from build123d import *

# Parameters (mm, degrees)
CUT_EXTRUDE1_START = -7
CUT_EXTRUDE1_DEPTH = 6


with BuildPart() as part:
    # Sketch3 → Revolve1 (revolve)
    with BuildSketch(Plane.XY, mode=Mode.PRIVATE) as revolve1_sk:
        Polygon((-7, 1.6), (6, 1.6), (6, 12), (15, 12), (15, 16), (-14, 16), (-14, 18), (-16, 18), (-16, 13), (-7, 13), align=None)
    revolve(revolve1_sk.sketch.rotate(Axis((0, 0, 0), (1, 0, 0)), 90), axis=Axis((0, 0, 0), (1, 0, 0)))

    # Sketch4 → Cut-Extrude1 (cut)
    with BuildSketch(Plane(origin=(0, 0, 0), x_dir=(0, 0, -1), z_dir=(1, 0, 0)).offset(CUT_EXTRUDE1_START)):
        Polygon((3.608439182, 6.25), (-3.608439182, 6.25), (-7.216878365, 0), (-3.608439182, -6.25), (3.608439182, -6.25), (7.216878365, 0), align=None)
    extrude(amount=CUT_EXTRUDE1_DEPTH, mode=Mode.SUBTRACT)


solid = part.part
Model file for the job. Use its own axes, mm. A direction names the side the tool comes from. Give positions to 0.01 mm unless a question says otherwise; leave off trailing zeros. Loops run counter-clockwise (first coordinate to the right, second up) from the corner with the lowest first, then second, coordinate; pieces in that order, holes last.
Item 1: Slice it at D-D (y = -5.5). Write the cut outline in (x, z), plus the area to 3 significant figures.
Check values:
outline: (-16, -17.14) - (-14, -17.14) - (-14, -15.02) - (15, -15.02) - (15, -10.67) - (6, -10.67) - (6, 10.67) - (15, 10.67) - (15, 15.02) - (-14, 15.02) - (-14, 17.14) - (-16, 17.14) - (-16, 11.78) - (-7, 11.78) - (-7, 4.04) - (-1, 4.04) - (-1, -4.04) - (-7, -4.04) - (-7, -11.78) - (-16, -11.78) - close
area: 488 mm2
Item 2: Slice it at B-B (x = -9.5). Write the cut outline in (y, z).
Check values:
outline: circle Ø32 at (0, 0); hole circle Ø26 at (0, 0)
Item 3: Slice it at A-A (z = 0). Write the cut outline in (x, y), plus the area to 3 significant figures.
Check values:
outline: (-16, -18) - (-14, -18) - (-14, -16) - (15, -16) - (15, -12) - (6, -12) - (6, -1.6) - (-1, -1.6) - (-1, -6.25) - (-7, -6.25) - (-7, -13) - (-16, -13) - close; (-16, 13) - (-7, 13) - (-7, 6.25) - (-1, 6.25) - (-1, 1.6) - (6, 1.6) - (6, 12) - (15, 12) - (15, 16) - (-14, 16) - (-14, 18) - (-16, 18) - close
area: 453 mm2
Item 4: Drill centre lines: line 1 along Y through (x, z) = (11, 0); line 2 along Y through (x, z) = (-12, 0); line 3 along X through (y, z) = (6.5, -10.5). Where is each one in solid material? Low to high.
Check values:
line 1: y = -16 to -12, 12 to 16
line 2: y = -16 to -13, 13 to 16
line 3: x = -7 to 15
Item 5: Mould opens along Z. For faces 4 (the face through (-7, -3, 6)), 5 (the face through (6, 0, -2)), 6 (the face through (-15.014, -12.165, -13.267)), 7 (the face through (-14, 11, 12)) say: +Z half, -Z half, draft (parallel to the pull), parting line (faces both ways), or undercut.
Check values:
face 4: undercut
face 5: undercut
face 6: parting line
face 7: draft
Item 6: Drop flat-ended pins along their axis: P1, Ø2, axis at y = 10.5, z = -4, coming from the +X side; P2, Ø2, axis at y = 2.5, z = 10.5, coming from the +X side; P3, Ø5, axis at x = -10.5, z = 13, coming from the -Y side; P4, Ø6, axis at x = -5, y = 2, coming from the +Z side. Give the stop position or say it passes through.
Check values:
P1: stops at x = 15
P2: stops at x = 6
P3: stops at y = -12.07
P4: stops at z = 16
Item 7: Slice it at C-C (z = -8). Write the cut outline in (x, y).
Check values:
outline: (-16, -16.12) - (-14, -16.12) - (-14, -13.86) - (15, -13.86) - (15, -8.94) - (6, -8.94) - (6, 8.94) - (15, 8.94) - (15, 13.86) - (-14, 13.86) - (-14, 16.12) - (-16, 16.12) - (-16, 10.25) - (-7, 10.25) - (-7, -10.25) - (-16, -10.25) - close
Item 8: Which spindle directions (+Z, -Z, +X, -X, +Y, -Y) get a long thin tool onto all of the face, cutting with end or side? Do faces 1 (the face through (10.563, -3.604, 11.446)), 2 (the face through (-4, -6.25, 0)), 3 (the face through (-16, -9.4, 9.2)). Say none if no direction does.
Check values:
face 1: +X
face 2: -X
face 3: +Z, -Z, -X, +Y, -Y
